For this review, take the finished solid that the model builds, in its own axes (mm). Round coordinates to 2 decimals unless told otherwise and drop trailing zeros. Loops run counter-clockwise (first coordinate to the right, second up) from the corner with the lowest first, then second, coordinate; pieces in that order, holes last.
1. Consider section A-A on x = 0. State the section outline as (y, z) points, then the cut area to 3 significant figures.
2. Clearance check with a flat-ended pin moving along its axis: pin 1 Ø6 at (y, z) = (-40, 0) entering from +X. State where the tip first meets the part, or that it passes through.
3. Consider section B-B on z = 0. State the section outline as (x, y) points (3 decimals), then the cut area to 3 significant figures.
4. Consider section D-D on x = -5.25. State the section outline as (y, z) points.
5. To check wall thickness, follow line 1 along Y through (x, z) = (0.25, 0); line 2 along Y through (x, z) = (0, -3.5); line 3 along X through (y, z) = (14, -1.75). State the ranges of each line that lie inside material, in increasing order.
6. Consider section C-C on y = -14. State the section outline as (x, z) points, then the cut area to 3 significant figures.
from build123d import *

# Parameters (mm, degrees)
CROQUIS1_W                         = 25.4
CROQUIS1_H                         = 100
SALIENTE_EXTRUIR1_DEPTH            = 6.35
TALADRO_DE_MARGEN_PARA_1_41_D      = 6.7564
TALADRO_ROSCADO_1_4_202_AT_2_COUNT = 2
TALADRO_ROSCADO_1_4_202_AT_2_PITCH = 80


with BuildPart() as part:
    # Croquis1 → Saliente-Extruir1 (new, symmetric)
    with BuildSketch(Plane.XY):
        Rectangle(CROQUIS1_W, CROQUIS1_H)
    extrude(amount=SALIENTE_EXTRUIR1_DEPTH, both=True)

    # Taladro de margen para 1/41 (through all)
    with Locations(Plane(origin=(-6.35, 0, 6.35), x_dir=(-1, 0, 0), z_dir=(0, 0, 1))):
        with Locations((-6.35, 14), (-6.35, -14)):
            Hole(TALADRO_DE_MARGEN_PARA_1_41_D / 2)

    # Croquis7 → Taladro roscado 1/4-202 (revolve, cut)
    with BuildSketch(Plane(origin=(-12.7, 40, 0), x_dir=(0, 0, 1), z_dir=(0, 1, 0))):
        Polygon((0, 0), (0, 25.4), (3.1877, 25.4), (2.5527, 24.765), (2.5527, 0.635), (3.1877, 0), align=None)
    taladro_roscado_1_4_202 = revolve(axis=Axis((-19.05, 40, 0), (1, 0, 0)), mode=Mode.SUBTRACT)

    # Taladro roscado 1/4-202 at 2: Taladro roscado 1/4-202 ×2
    with Locations(*[(0, -i * TALADRO_ROSCADO_1_4_202_AT_2_PITCH, 0) for i in range(1, TALADRO_ROSCADO_1_4_202_AT_2_COUNT)]):
        add(taladro_roscado_1_4_202, mode=Mode.SUBTRACT)


solid = part.part
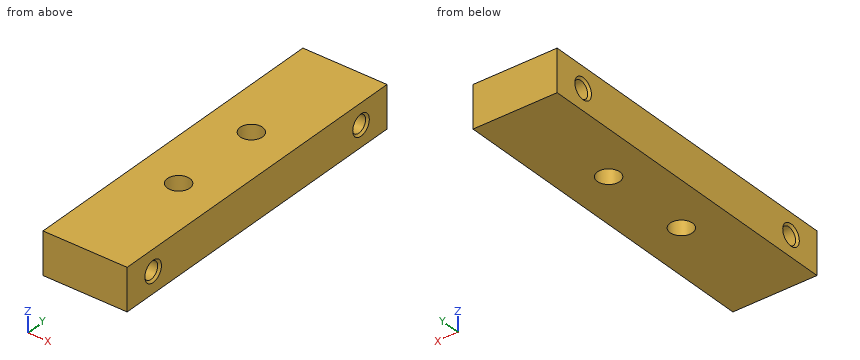
Resolved:
1. outline: (-50, -6.35) - (-17.38, -6.35) - (-17.38, 6.35) - (-50, 6.35) - close; (-10.62, -6.35) - (10.62, -6.35) - (10.62, 6.35) - (-10.62, 6.35) - close; (17.38, -6.35) - (50, -6.35) - (50, 6.35) - (17.38, 6.35) - close; hole circle Ø5.11 at (-40, 0); hole circle Ø5.11 at (40, 0)
1. area: 1,060 mm2
2. pin 1: stops at x = 12.51
3. outline: (-12.7, -50) - (12.7, -50) - (12.7, -43.188) - (12.065, -42.553) - (-12.065, -42.553) - (-12.7, -43.188) - close; (-12.7, -36.812) - (-12.065, -37.447) - (12.065, -37.447) - (12.7, -36.812) - (12.7, 36.812) - (12.065, 37.447) - (-12.065, 37.447) - (-12.7, 36.812) - close; (-12.7, 43.188) - (-12.065, 42.553) - (12.065, 42.553) - (12.7, 43.188) - (12.7, 50) - (-12.7, 50) - close; hole circle Ø6.756 at (0, -14); hole circle Ø6.756 at (0, 14)
3. area: 2,210 mm2
4. outline: (-50, -6.35) - (50, -6.35) - (50, 6.35) - (-50, 6.35) - close; hole circle Ø5.11 at (-40, 0); hole circle Ø5.11 at (40, 0)
5. line 1: y = -50 to -42.55, -37.45 to -17.37, -10.63 to 10.63, 17.37 to 37.45, 42.55 to 50
5. line 2: y = -50 to -17.38, -10.62 to 10.62, 17.38 to 50
5. line 3: x = -12.7 to -3.38, 3.38 to 12.7
6. outline: (-12.7, -6.35) - (-3.38, -6.35) - (-3.38, 6.35) - (-12.7, 6.35) - close; (3.38, -6.35) - (12.7, -6.35) - (12.7, 6.35) - (3.38, 6.35) - close
6. area: 237 mm2
